Verification items for the finished model (mm, model axes). A direction names the side the tool comes from. Round coordinates to 2 decimals unless told otherwise and drop trailing zeros. Write each loop counter-clockwise with the first axis right and the second up, starting at its lowest first coordinate (ties: lowest second). Pieces come first, ordered by that corner, then holes. Notation, with made-up numbers: (-11, 36.5) - (16, 36.5) arc R17 ccw to (16, 50.5) - close; hole circle Ø4 at (3, 45.5). An arc over 180 degrees is marked (long way). Answer as a JSON object with one key per item and string values.
```python
from build123d import *

# Parameters (mm, degrees)
EXTRUDE_1_DEPTH     = 10
CUT_EXTRUDE_1_DEPTH = 5


with BuildPart() as part:
    # 草圖2 → 填料-伸長1 (new body)
    with BuildSketch(Plane.XY):
        Polygon((-40, 7.5), (-38, 7.5), (-38, -7.5), (-40, -7.5), (-40, -10), (40, -10), (40, 10), (-40, 10), align=None)
    extrude(amount=EXTRUDE_1_DEPTH)

    # 草圖3 → 除料-伸長1 (cut)
    with BuildSketch(Plane.XY.offset(10)):
        Polygon((2.679491924, 10), (14.226497308, -10), (37.320508076, -10), (25.773502692, 10), align=None)
    extrude(amount=-CUT_EXTRUDE_1_DEPTH, mode=Mode.SUBTRACT)


solid = part.part
```
Q1. Section check B-B, the plane z = 1. Record the cut outline in (x, y).
Geometry check:
{"outline": "(-40, -10) - (40, -10) - (40, 10) - (-40, 10) - (-40, 7.5) - (-38, 7.5) - (-38, -7.5) - (-40, -7.5) - close"}
Q2. Release check for a two-part mould opening along X. For faces 1 (the flat face through (31.63, -0.14, 7.54)), 2 (the flat face through (-40, 9, 5)), 3 (the flat face through (-9, -10, 5)), 4 (the flat face through (40, 0, 5)) record: released by +X, released by -X, zero draft, split by the parting line, or undercut.
Geometry check:
{"face 1": "undercut", "face 2": "released by -X", "face 3": "zero draft", "face 4": "released by +X"}
Q3. Gauge pin test, flat end, axial feed: P1, Ø3, axis at y = 1, z = 6.5, coming from the -X side. Record the tip position at first contact, or that the pin passes through.
Geometry check:
{"P1": "stops at x = -38"}
Q4. Section check D-D, the plane x = 21. Record the cut outline in (y, z), then the cut area to 3 significant figures.
Geometry check:
{"outline": "(-10, 0) - (10, 0) - (10, 5) - (-10, 5) - close", "area": "100 mm2"}
Q5. Section check C-C, the plane y = -8.5. Record the cut outline in (x, z), then the cut area to 3 significant figures.
Geometry check:
{"outline": "(-40, 0) - (40, 0) - (40, 10) - (36.45, 10) - (36.45, 5) - (13.36, 5) - (13.36, 10) - (-40, 10) - close", "area": "685 mm2"}
Q6. Set-up check for faces 5 (the flat face through (20, 0, 5)), 6 (the flat face through (8.37, 0.14, 7.54)), 7 (the flat face through (-38, 0, 5)): record each of +Z, -Z, +X, -X, +Y, -Y from which the full face is reachable in a straight line by a thin tool's end or side.
Geometry check:
{"face 5": "+Z", "face 6": "+Z, +Y", "face 7": "+Z, -Z, -X"}
Q7. Section check A-A, the plane z = 6. Record the cut outline in (x, y).
Geometry check:
{"outline": "(-40, -10) - (14.23, -10) - (2.68, 10) - (-40, 10) - (-40, 7.5) - (-38, 7.5) - (-38, -7.5) - (-40, -7.5) - close; (25.77, 10) - (37.32, -10) - (40, -10) - (40, 10) - close"}
Q8. Material ranges on line 1 along X through (y, z) = (4.5, 6.25); line 2 along X through (y, z) = (0.25, 6.75); line 3 along X through (y, z) = (6.75, 4.25), recorded low to high. Write a range as [from, to].
Geometry check:
{"line 1": "x = [-38, 5.85], [28.95, 40]", "line 2": "x = [-38, 8.31], [31.4, 40]", "line 3": "x = [-38, 40]"}
